The listing builds one solid part. Answer for the finished solid, in the listing's coordinates (mm). Face numbers are marked on the shaded views. A direction names the side the tool comes from. Round coordinates to 2 decimals unless told otherwise and drop trailing zeros. Loops run counter-clockwise (first coordinate to the right, second up) from the corner with the lowest first, then second, coordinate; pieces in that order, holes last. Notation, with made-up numbers: (55, 28) -> (105, 28) arc R14 cw to (105, 53) -> close; hole circle Ø11 at (42, 83). An arc over 180 degrees is marked (long way). Use a Markdown table: item, result. Add a question column.
Q1. For a pull along Y with two mould halves and no side action, classify the marked faces 3, 4 and 5 as released by +Y, released by -Y, zero draft, split by the parting line, or undercut.
Q2. Section A-A on z = -16.25 is taken. Give the vertices of the cut face in (x, y), then the cut area to 3 significant figures.
Q3. Consider line 1 (Y direction, x = 1, z = -4.25); line 2 (Z direction, x = 2, y = 9). Determine where each line is inside the solid, lowest interval first.
Q4. Which of the six approach directions +Z, -Z, +X, -X, +Y, -Y give full straight-line access (tool end or side, diameter ignored) to the marked faces 1 and 2?
Q5. Given pin 1 Ø3 at (x, y) = (5, 10) entering from +Z, flat-ended and moving along its own axis, determine where the tip first touches the part or whether it passes through.
Q6. Section B-B on x = 4 is taken. Give the vertices of the cut face in (y, z).
Q7. Section C-C on y = 19.5 is taken. Give the vertices of the cut face in (x, z), then the cut area to 3 significant figures.
Autodesk Inventor part; units mm, degrees
ref_plane "YZ Plane" through (0, 0, 0) normal (1, 0, 0) x (0, 1, 0)
ref_plane "XZ Plane" through (0, 0, 0) normal (0, 1, 0) x (-1, 0, 0)
ref_plane "XY Plane" through (0, 0, 0) normal (0, 0, 1) x (1, 0, 0)
sketch "Sketch1" plane through (0, 0, 0) normal (1, 0, 0) x (0, 1, 0)
  line L0 (0, 0) -> (20, 0) construction
  line L1 (20, 0) -> (20, -21.5)
  line L2 (20, -21.5) -> (0, -21.5)
  line L3 (0, -21.5) -> (0, 0)
  line L4 (20, 0) -> (26.35, 0)
  line L5 (26.35, 0) -> (26.35, -27.85)
  line L6 (-6.35, -27.85) -> (-6.35, 0)
  line L7 (-6.35, 0) -> (0, 0)
  line L8 (26.35, -27.85) -> (-6.35, -27.85)
  dimension "d0" = 20
  dimension "d1" = 21.5
  dimension "d4" = 6.35
  dimension "d23" = 6.35
  dimension "d24" = 6.35
extrude "Extrusion1" add sketch "Sketch1" along normal blind 6.35
properties part number "Main"
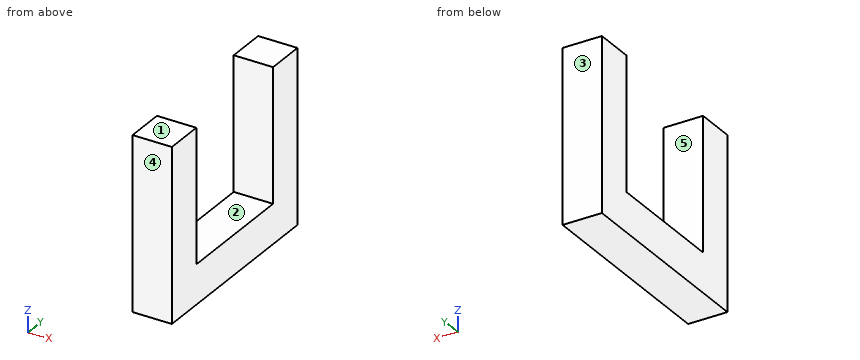
Checked values:
| question | item | result |
|---|---|---|
| 1 | face 3 | released by +Y |
| 1 | face 4 | released by -Y |
| 1 | face 5 | undercut |
| 2 | outline | (0, -6.35) -> (6.35, -6.35) -> (6.35, 0) -> (0, 0) -> close; (0, 20) -> (6.35, 20) -> (6.35, 26.35) -> (0, 26.35) -> close |
| 2 | area | 80.6 mm2 |
| 3 | line 1 | y = -6.35 to 0, 20 to 26.35 |
| 3 | line 2 | z = -27.85 to -21.5 |
| 4 | face 1 | +Z, +X, -X, +Y, -Y |
| 4 | face 2 | +Z, +X, -X |
| 5 | pin 1 | stops at z = -21.5 |
| 6 | outline | (-6.35, -27.85) -> (26.35, -27.85) -> (26.35, 0) -> (20, 0) -> (20, -21.5) -> (0, -21.5) -> (0, 0) -> (-6.35, 0) -> close |
| 7 | outline | (0, -27.85) -> (6.35, -27.85) -> (6.35, -21.5) -> (0, -21.5) -> close |
| 7 | area | 40.3 mm2 |
